from build123d import *

# Parameters (mm, degrees)
F0_W      = 38.1
F0_H      = 38.1
F1_DEPTH  = 38.1
F6_DEPTH  = 38.1
F8_DEPTH  = 38.1
F9_W      = 25.4
F9_H      = 7.62
F10_DEPTH = 38.1


with BuildPart() as f1:
    # F0 (on Front) → F1 (new body)
    with BuildSketch(Plane.XZ):
        with Locations((19.05, 19.05)):
            Rectangle(F0_W, F0_H)
    extrude(amount=F1_DEPTH)

    # F5 (on offset) → F6 (cut)
    with BuildSketch(Plane.YZ.offset(38.1)):
        Polygon((-6.35, 38.1), (-31.75, 38.1), (-26.67, 15.875), (-21.59, 28.575), (-16.51, 28.575), (-11.43, 15.875), align=None)
        Polygon((-19.05, 15.875), (-25.4, 0), (-12.7, 0), align=None)
        Polygon((-31.75, 0), (-38.1, 38.1), (-38.1, 0), align=None)
        Polygon((0, 0), (0, 38.1), (-6.35, 0), align=None)
    extrude(amount=-F6_DEPTH, mode=Mode.SUBTRACT)

    # F7 (on offset) → F8 (cut)
    with BuildSketch(Plane.XZ.offset(38.1)):
        Polygon((0, 38.1), (0, 0), (6.35, 38.1), align=None)
        Polygon((25.4, 38.1), (12.7, 38.1), (19.05, 22.225), align=None)
        Polygon((31.75, 38.1), (38.1, 0), (38.1, 38.1), align=None)
        Polygon((11.43, 21.636641), (6.35, 0), (31.75, 0), (26.67, 22.225), (21.59, 9.525), (16.51, 9.525), align=None)
    extrude(amount=-F8_DEPTH, mode=Mode.SUBTRACT)

    # F9 (on offset) → F10 (cut)
    with BuildSketch(Plane.XY.offset(38.1)):
        with Locations((25.4, -11.43)):
            Rectangle(F9_W, F9_H)
        with Locations((12.7, -26.67)):
            Rectangle(F9_W, F9_H)
    extrude(amount=-F10_DEPTH, mode=Mode.SUBTRACT)


solid = f1.part
Input: part model. Units: mm. Frame: model coordinates. A direction names the side the tool comes from. Give positions to 0.01 mm unless a question says otherwise; leave off trailing zeros. Order: outer loops, then holes, each group sorted by start corner. A loop starts at its lowest first (then second) coordinate and runs counter-clockwise, first axis right, second up. Notation, with made-up numbers: M -5,-22.75 L 36,-22.75 A11 cw 36,-8.75 Z; hole C 51,72 d3. An arc over 180 degrees is marked long. Answer as a JSON object with one key per item and string values.
1. Cut plane D-D, the plane z = 31. Output: boundary loops of the cut face in (x, y).
Result sheet:
{"outline": "M 5.17,-36.92 L 15.54,-36.92 L 15.54,-30.48 L 5.17,-30.48 Z; M 5.17,-7.97 L 12.7,-7.97 L 12.7,-7.62 L 15.54,-7.62 L 15.54,-1.18 L 5.17,-1.18 Z; M 22.56,-36.92 L 32.93,-36.92 L 32.93,-30.13 L 25.4,-30.13 L 25.4,-30.48 L 22.56,-30.48 Z; M 22.56,-7.62 L 32.93,-7.62 L 32.93,-1.18 L 22.56,-1.18 Z"}
2. Cut plane A-A, the plane x = 9. Output: boundary loops of the cut face in (y, z) (3 decimals).
Result sheet:
{"outline": "M -38.1,38.1 L -33.631,11.287 L -30.48,11.287 L -30.48,32.544 L -31.75,38.1 Z; M -22.86,11.287 L -20.885,11.287 L -19.05,15.875 L -17.215,11.287 L -4.469,11.287 L 0,38.1 L -6.35,38.1 L -11.43,15.875 L -16.51,28.575 L -21.59,28.575 L -22.86,25.4 Z"}
3. Ray query, line 1 (X direction, y = -5, z = 13.5); line 2 (Y direction, x = 11.5, z = 23); line 3 (Y direction, x = 31.5, z = 7.5). Return the intervals inside material, ascending. Write a range as [from, to].
Result sheet:
{"line 1": "[2.25, 9.52], [14.84, 23.18], [28.66, 35.85]", "line 2": "[-35.58, -30.48], [-22.86, -14.28], [-9.8, -2.52]", "line 3": "[-33, -22.4], [-15.7, -15.24], [-7.62, -5.1]"}
4. Cut plane B-B, the plane z = 5. Output: boundary loops of the cut face in (x, y), and give its area (3 significant figures).
Result sheet:
{"outline": "M 0.83,-32.58 L 7.52,-32.58 L 7.52,-30.48 L 0.83,-30.48 Z; M 0.83,-14.7 L 7.52,-14.7 L 7.52,-5.52 L 0.83,-5.52 Z; M 30.61,-32.58 L 37.27,-32.58 L 37.27,-23.4 L 30.61,-23.4 Z; M 30.61,-7.62 L 37.27,-7.62 L 37.27,-5.52 L 30.61,-5.52 Z", "area": "151 mm²"}
5. Reachability of faces 1 (the flat face through (15.83, -4.71, 30.27)), 2 (the flat face through (19, -22, 9.525)), 3 (the flat face through (19.06, -18.044, 13.361)), 4 (the flat face through (11, -19, 28.575)) from +Z, -Z, +X, -X, +Y, -Y: full face, straight path, thin tool, end or side. Return the list, or none.
Result sheet:
{"face 1": "+Z, +Y, -Y", "face 2": "-Z, +Y, -Y", "face 3": "-Z, +X, -X", "face 4": "+Z, +X, -X"}
6. Cut plane C-C, the plane y = -32.5. Output: boundary loops of the cut face in (x, z) (3 decimals), and give its area (3 significant figures).
Result sheet:
{"outline": "M 0.75,4.5 L 7.407,4.5 L 11.43,21.637 L 16.51,9.525 L 21.59,9.525 L 26.67,22.225 L 30.721,4.5 L 37.35,4.5 L 31.75,38.1 L 25.4,38.1 L 19.05,22.225 L 12.7,38.1 L 6.35,38.1 Z", "area": "731 mm²"}
7. Pull-direction query (Y, two-part tool) for faces 5 (the flat face through (22.2, -33.5, 30.1)), 6 (the flat face through (24.7, -15.24, 18.1)), 7 (the flat face through (19.32, -3.13, 19.32)); classes: +Y half, -Y half, draft (parallel to the pull), parting line (faces both ways), or undercut.
Result sheet:
{"face 5": "draft", "face 6": "undercut", "face 7": "+Y half"}
8. First-contact query: P1, Ø4, axis at x = 30, y = -18, coming from the +Z side (3 decimals); P2, Ø12.5, axis at x = 23.5, z = 20, coming from the -Y side (3 decimals); P3, Ø3.5, axis at y = -9.5, z = 23, coming from the +X side; P4, Ø2, axis at x = 24, y = -26, coming from the +Z side. Flat tips, straight axial feed; report the tip coordinate or a pass-through.
Result sheet:
{"P1": "z = 28.575", "P2": "y = -36.125", "P3": "x = 12.7", "P4": "through"}
